Read the model definition and answer for the solid it produces. Units are mm, in the model's axes. A direction names the side the tool comes from. Coordinates: 2 decimals unless noted, no trailing zeros. Write each loop counter-clockwise with the first axis right and the second up, starting at its lowest first coordinate (ties: lowest second). Pieces come first, ordered by that corner, then holes. Notation, with made-up numbers: M 28.25,34.25 L 49.25,34.25 A12 cw 49.25,39.25 Z; hole C 84,67.5 d3. An arc over 180 degrees is marked long. Use a Markdown table: item, result. Add a question column.
from build123d import *

# Parameters (mm, degrees)
ESQUISSE1_R             = 43
ESQUISSE1_R_2           = 36
BASE_EXTRUSION_DEPTH    = 50
ESQUISSE2_R             = 2
ENL_V_MAT_EXTRU_1_DEPTH = 81.120222166


with BuildPart() as part:
    # Esquisse1 → Base-Extrusion (new body)
    with BuildSketch(Plane.XY):
        with Locations((0, 2.5)):
            Circle(ESQUISSE1_R)
        Circle(ESQUISSE1_R_2, mode=Mode.SUBTRACT)
    extrude(amount=BASE_EXTRUSION_DEPTH)

    # Esquisse2 → Enl_v. mat.-Extru.1 (cut, through all)
    with BuildSketch(Plane(origin=(0, 0, 0), x_dir=(1, 0, 0), z_dir=(0, 1, 0))):
        with Locations(Location((0, -8, 0), (0, 0, 270))):
            Circle(ESQUISSE2_R)
        with Locations(Location((0, -16, 0), (0, 0, 270))):
            Circle(ESQUISSE2_R)
        with Locations(Location((0, -24, 0), (0, 0, 270))):
            Circle(ESQUISSE2_R)
        with Locations(Location((0, -32, 0), (0, 0, 270))):
            Circle(ESQUISSE2_R)
        with Locations(Location((0, -40, 0), (0, 0, 270))):
            Circle(ESQUISSE2_R)
        with Locations((0, 92)):
            Circle(ESQUISSE2_R)
        with Locations((0, 84)):
            Circle(ESQUISSE2_R)
        with Locations((0, 76)):
            Circle(ESQUISSE2_R)
        with Locations((0, 68)):
            Circle(ESQUISSE2_R)
        with Locations((0, 60)):
            Circle(ESQUISSE2_R)
        with Locations((0, 192)):
            Circle(ESQUISSE2_R)
        with Locations((0, 184)):
            Circle(ESQUISSE2_R)
        with Locations((0, 176)):
            Circle(ESQUISSE2_R)
        with Locations((0, 168)):
            Circle(ESQUISSE2_R)
        with Locations((0, 160)):
            Circle(ESQUISSE2_R)
        with Locations((0, 292)):
            Circle(ESQUISSE2_R)
        with Locations((0, 284)):
            Circle(ESQUISSE2_R)
        with Locations((0, 276)):
            Circle(ESQUISSE2_R)
        with Locations((0, 268)):
            Circle(ESQUISSE2_R)
        with Locations((0, 260)):
            Circle(ESQUISSE2_R)
        with Locations((0, 392)):
            Circle(ESQUISSE2_R)
        with Locations((0, 384)):
            Circle(ESQUISSE2_R)
        with Locations((0, 376)):
            Circle(ESQUISSE2_R)
        with Locations((0, 368)):
            Circle(ESQUISSE2_R)
        with Locations((0, 360)):
            Circle(ESQUISSE2_R)
    extrude(amount=-ENL_V_MAT_EXTRU_1_DEPTH, mode=Mode.SUBTRACT)


solid = part.part
Item 1: Find section C-C on z = 19.5. Give the vertices of the cut face in (x, y), then the cut area to 3 significant figures.
Item 2: Each of these flat-tipped pins is pushed along its axis until it touches: pin 1 (2.5 mm diameter, centred on x = 0, z = 40, fed in from +Y); pin 2 (2 mm diameter, centred on x = -12.5, z = 5, fed in from +Y); pin 3 (1.5 mm diameter, centred on y = 31, z = 39.5, fed in from +X). Where does it stop, or does it pass through?
Item 3: For faces 5 (the cylindrical face through (-1.774, -38.191, 16.923)), 6 (the flat face through (-13, 35, 0)), determine the directions among +Z, -Z, +X, -X, +Y, -Y from which every point of the face is accessible in a straight line to the end or side of a thin tool.
Item 4: Determine the mould class of faces 1 (the cylindrical face through (-4.686, 35.694, 24.65)), 2 (the flat face through (-13, 35, 50)), 3 (the cylindrical face through (-0.766, -38.191, 33.847)), 4 (the cylindrical face through (-31.693, 31.561, 24.65)) for opening direction X: pulls with the +X half, pulls with the -X half, needs draft (parallel to the pull), parting line crosses it, or undercut.
Item 5: Find section A-A on x = 0. Give the vertices of the cut face in (y, z).
Item 6: Find section D-D on x = -13. Give the vertices of the cut face in (y, z).
Item 7: Consider probe 1 along Z at (x, y) = (0, -37.6); probe 2 along Y at (x, z) = (-31, 38.5); probe 3 along Y at (x, z) = (-13.5, 11). Determine where each line is inside the solid, lowest interval first.
Item 8: Find section B-B on y = -3. Give the vertices of the cut face in (x, z), then the cut area to 3 significant figures.
Geometry says:
| question | item | result |
|---|---|---|
| 1 | outline | C 0,2.5 d86; hole C 0,0 d72 |
| 1 | area | 1,740 mm2 |
| 2 | pin 1 | stops at y = 45.5 |
| 2 | pin 2 | stops at y = 43.93 |
| 2 | pin 3 | stops at x = 32.85 |
| 3 | face 5 | -Y |
| 3 | face 6 | -Z, +X, -X, +Y, -Y |
| 4 | face 1 | undercut |
| 4 | face 2 | needs draft |
| 4 | face 3 | undercut |
| 4 | face 4 | parting line crosses it |
| 5 | outline | M -40.5,0 L -36,0 L -36,6 L -40.5,6 Z; M -40.5,10 L -36,10 L -36,14 L -40.5,14 Z; M -40.5,18 L -36,18 L -36,22 L -40.5,22 Z; M -40.5,26 L -36,26 L -36,30 L -40.5,30 Z; M -40.5,34 L -36,34 L -36,38 L -40.5,38 Z; M -40.5,42 L -36,42 L -36,50 L -40.5,50 Z; M 36,0 L 45.5,0 L 45.5,50 L 36,50 Z |
| 6 | outline | M -38.49,0 L -33.57,0 L -33.57,50 L -38.49,50 Z; M 33.57,0 L 43.49,0 L 43.49,50 L 33.57,50 Z |
| 7 | probe 1 | z = 0 to 6, 10 to 14, 18 to 22, 26 to 30, 34 to 38, 42 to 50 |
| 7 | probe 2 | y = -27.3 to -18.3, 18.3 to 32.3 |
| 7 | probe 3 | y = -38.33 to -33.37, 33.37 to 43.33 |
| 8 | outline | M -42.65,0 L -35.87,0 L -35.87,50 L -42.65,50 Z; M 35.87,0 L 42.65,0 L 42.65,50 L 35.87,50 Z |
| 8 | area | 677 mm2 |
